```python
from build123d import *

# Parameters (mm, degrees)
F1_DEPTH = 6
F3_DEPTH = 6
F5_DEPTH = 6


with BuildPart() as f1:
    # F0 (on Top) → F1 (new body)
    with BuildSketch(Plane.XY):
        with BuildLine():
            Line((64, 0), (0, 0))
            Line((0, 0), (0, -25))
            Line((0, -25), (64, -25))
            Line((64, -25), (64, -19))
            Line((64, -19), (44, -19))
            ThreePointArc((44, -19), (37.5, -12.5), (44, -6))
            Line((44, -6), (64, -6))
            Line((64, -6), (64, 0))
        make_face()
    extrude(amount=F1_DEPTH)

    # F2 (on face) → F3 (join)
    with BuildSketch(Plane(origin=(0, 0, 0), x_dir=(0, -1, 0), z_dir=(-1, 0, 0))):
        with BuildLine():
            Line((0, 0), (25, 0))
            Line((25, 0), (25, 18))
            ThreePointArc((25, 18), (12.5, 5.5), (0, 18))
            Line((0, 18), (0, 0))
        make_face()
        with BuildLine():
            ThreePointArc((0, 18), (12.5, 5.5), (25, 18))
            Line((25, 18), (19, 18))
            ThreePointArc((19, 18), (12.5, 11.5), (6, 18))
            Line((6, 18), (0, 18))
        make_face()
        with BuildLine():
            Line((19, 18), (25, 18))
            ThreePointArc((25, 18), (12.5, 30.5), (0, 18))
            Line((0, 18), (6, 18))
            ThreePointArc((6, 18), (12.5, 24.5), (19, 18))
        make_face()
    extrude(amount=F3_DEPTH)

    # F4 (on face) → F5 (join)
    with BuildSketch(Plane(origin=(0, 0, 0), x_dir=(-1, 0, 0), z_dir=(0, 1, 0))):
        with BuildLine():
            Line((6, -12.0803898498), (6, 5.9196101502))
            Line((6, 5.9196101502), (-19, 5.9196101502))
            Line((-19, 5.9196101502), (-19, -12.0803898498))
            ThreePointArc((-19, -12.0803898498), (-6.5, 0.4196101502), (6, -12.0803898498))
        make_face()
        with BuildLine():
            ThreePointArc((-19, -12.0803898498), (-6.5, -24.5803898498), (6, -12.0803898498))
            Line((6, -12.0803898498), (0, -12.0803898498))
            ThreePointArc((0, -12.0803898498), (-6.5, -18.5803898498), (-13, -12.0803898498))
            Line((-13, -12.0803898498), (-19, -12.0803898498))
        make_face()
        with BuildLine():
            Line((0, -12.0803898498), (6, -12.0803898498))
            ThreePointArc((6, -12.0803898498), (-6.5, 0.4196101502), (-19, -12.0803898498))
            Line((-19, -12.0803898498), (-13, -12.0803898498))
            ThreePointArc((-13, -12.0803898498), (-6.5, -5.5803898498), (0, -12.0803898498))
        make_face()
    extrude(amount=-F5_DEPTH)


solid = f1.part
```
Input: part model. Units: mm. Frame: model coordinates. A direction names the side the tool comes from. Give positions to 0.01 mm unless a question says otherwise; leave off trailing zeros. Order: outer loops, then holes, each group sorted by start corner. A loop starts at its lowest first (then second) coordinate and runs counter-clockwise, first axis right, second up. Notation, with made-up numbers: M 12,36 L 22,36 A16 ccw 22,62 Z; hole C 75,-7 d2. An arc over 180 degrees is marked long. One line per question, with ' | ' between items. Start each with the question number.
1. Section query A-A (x = 45). Return the cut outline in (y, z), and give its area (3 significant figures).
2. Section query C-C (z = 5). Return the cut outline in (x, y).
3. Material intervals for probe 1 along Z at (x, y) = (-3.3, -12.5); probe 2 along Z at (x, y) = (6.5, -4.5); probe 3 along X at (y, z) = (-23.25, 18), sorted ascending. Write a range as [from, to].
4. Pull-direction query (Y, two-part tool) for faces 1 (the face through (-2.958, -9.006, 23.481)), 2 (the face through (6.775, -2.958, -24.577)), 3 (the face through (-2.958, -12.775, 30.497)), 4 (the face through (37.5, -12.6, 3)); classes: released by +Y, released by -Y, zero draft, split by the parting line, or undercut.
5. Access query for faces 5 (the face through (24, -12, 6)), 6 (the face through (54, -19, 3)), 7 (the face through (3.501, -2.958, -6.314)), 8 (the face through (19, -3, -6)), 9 (the face through (1, -6, -7)). Directions: +Z, -Z, +X, -X, +Y, -Y. A direction counts if a zero-diameter tool reaches every point of the face in a straight line with its end or side. Return the directions, or none.
6. Section query D-D (y = -4.75). Return the cut outline in (x, z), and give its area (3 significant figures).
7. First-contact query: pin 1 Ø1 at (x, y) = (20.5, -12) entering from +Z; pin 2 Ø6.5 at (y, z) = (-3, -8) entering from +X; pin 3 Ø6 at (x, y) = (44.5, -4) entering from -Z; pin 4 Ø8 at (x, z) = (6.5, -12.08) entering from -Y. Flat tips, straight axial feed; report the tip coordinate or a pass-through.
8. Section query B-B (y = -12.5). Return the cut outline in (x, z), and give its area (3 significant figures).
Here are the results:
1) outline: M -25,0 L -19,0 L -19,6 L -25,6 Z; M -6,0 L 0,0 L 0,6 L -6,6 Z | area: 72.0 mm²
2) outline: M -6,-25 L 64,-25 L 64,-19 L 44,-19 A6.5 cw 44,-6 L 64,-6 L 64,0 L -6,0 Z
3) probe 1: [0, 11.5], [24.5, 30.5] | probe 2: [-24.58, -18.58], [-5.58, 6] | probe 3: [-6, 0]
4) face 1: undercut | face 2: zero draft | face 3: split by the parting line | face 4: undercut
5) face 5: +Z, +X, +Y, -Y | face 6: +Z, -Z, +X | face 7: +Y, -Y | face 8: -Z, +X, +Y, -Y | face 9: -Z, +X, -X, -Y
6) outline: M -6,-12.08 A12.5 ccw 19,-12.08 L 19,0 L 64,0 L 64,6 L 0,6 L 0,27.81 L -6,27.81 Z; hole C 6.5,-12.08 d13 | area: 966 mm²
7) pin 1: z = 6 | pin 2: x = 19 | pin 3: z = 0 | pin 4: through
8) outline: M -6,0 L 37.5,0 L 37.5,6 L 0,6 L 0,11.5 L -6,11.5 Z; M -6,24.5 L 0,24.5 L 0,30.5 L -6,30.5 Z | area: 330 mm²
